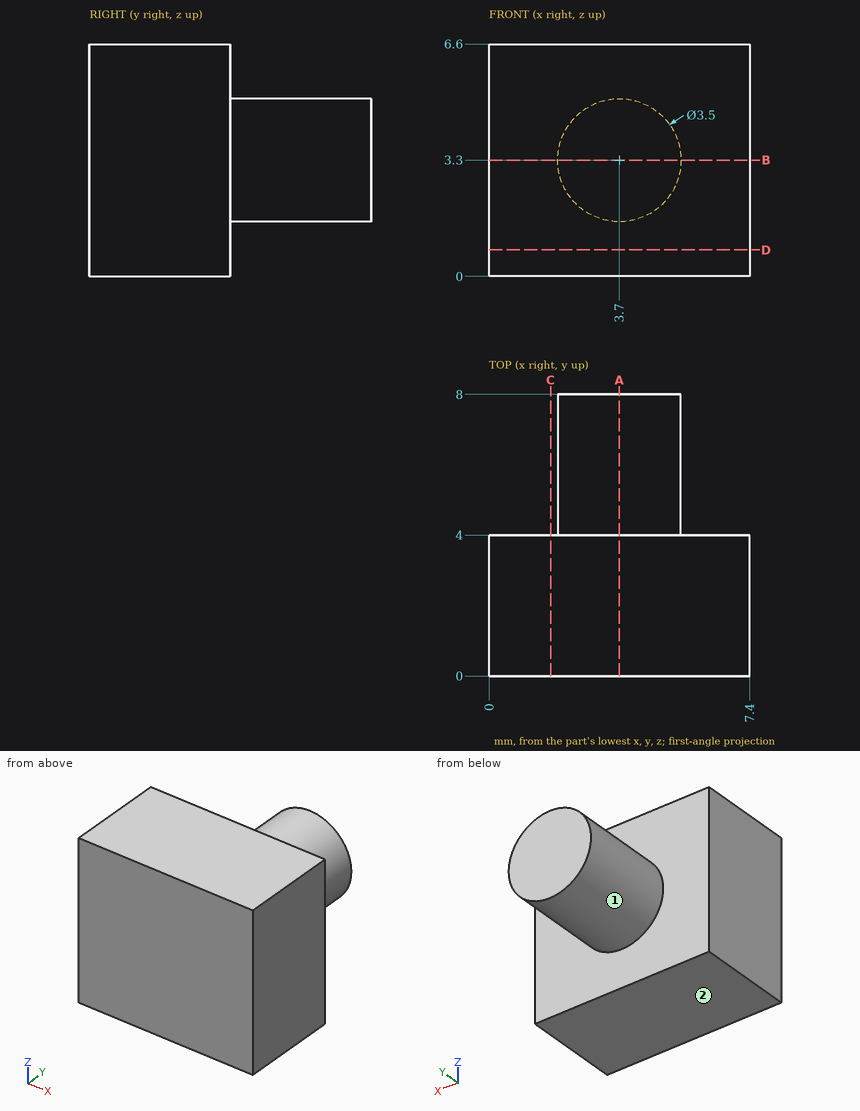
Drawing for the job (mm, zero at the part's lowest x, y, z). A direction names the side the tool comes from. Give positions to 0.01 mm unless a question says otherwise; leave off trailing zeros. Order: outer loops, then holes, each group sorted by start corner. A loop starts at its lowest first (then second) coordinate and runs counter-clockwise, first axis right, second up. Notation, with made-up numbers: (-12, 29.5) - (37, 29.5) arc R14 ccw to (37, 44.5) - close; hole circle Ø9 at (-7.5, 58). An arc over 180 degrees is marked (long way). Use one line per item in the form item = value.
Item 1: Pin check, flat tip, straight feed: pin 1 Ø1.5 at (y, z) = (6.5, 1) entering from +X. Stop position of the tip, or through.
Solution:
pin_1 = 4.51
Item 2: Slice it at D-D on z = 0.75. Give the cut face in (x, y).
Solution:
outline = (0, 0) - (7.4, 0) - (7.4, 4) - (0, 4) - close
Item 3: Slice it at A-A on x = 3.7. Give the cut face in (y, z).
Solution:
outline = (0, 0) - (4, 0) - (4, 1.55) - (8, 1.55) - (8, 5.05) - (4, 5.05) - (4, 6.6) - (0, 6.6) - close
Item 4: Slice it at C-C on x = 1.75. Give the cut face in (y, z).
Solution:
outline = (0, 0) - (4, 0) - (4, 6.6) - (0, 6.6) - close
Item 5: Which spindle directions (+Z, -Z, +X, -X, +Y, -Y) get a long thin tool onto all of the face, cutting with end or side? Do the marked faces 1 and 2. Say none if no direction does.
Solution:
face_1 = +Y
face_2 = -Z, +X, -X, +Y, -Y
Item 6: Slice it at B-B on z = 3.3. Give the cut face in (x, y), and give its area (3 significant figures).
Solution:
outline = (0, 0) - (7.4, 0) - (7.4, 4) - (5.45, 4) - (5.45, 8) - (1.95, 8) - (1.95, 4) - (0, 4) - close
area = 43.6 mm2
Item 7: Probe probe 1 along Y at (x, z) = (6, 3.75); probe 2 along X at (y, z) = (6.5, 1.75); probe 3 along Z at (x, y) = (2.5, 7.75). List the from-to ranges inside material, lowest first. Write a range as from..to.
Solution:
probe_1 = 0..4
probe_2 = 2.89..4.51
probe_3 = 2.03..4.57
